```python
from build123d import *

# Parameters (mm, degrees)
F1_DEPTH = 6.0198
F3_DEPTH = 6.0198
F4_R     = 7.62
F5_R     = 1.27


with BuildPart() as f1:
    # F0 (on Top) → F1 (new body)
    with BuildSketch(Plane.XY):
        with BuildLine():
            ThreePointArc((-5.588, -10.4775), (0, 11.8745), (5.588, -10.4775))
            Line((5.588, -10.4775), (5.588, -17.0815))
            Line((5.588, -17.0815), (19.1516, -17.0815))
            Line((19.1516, -17.0815), (19.1516, 21.4503))
            Line((19.1516, 21.4503), (-6.5024, 38.3413))
            ThreePointArc((-6.5024, 38.3413), (-15.638779, 32.001463), (-19.1516, 21.4503))
            Line((-19.1516, 21.4503), (-19.1516, -17.0815))
            Line((-19.1516, -17.0815), (-5.588, -17.0815))
            Line((-5.588, -17.0815), (-5.588, -10.4775))
        make_face()
    extrude(amount=F1_DEPTH)

    # F2 (on face) → F3 (cut, through all)
    with BuildSketch(Plane.XY.offset(6.0198)):
        with BuildLine():
            ThreePointArc((-6.444942, 33.269299), (-11.999418, 28.483341), (-14.0716, 21.4503))
            ThreePointArc((-14.0716, 21.4503), (-11.5316, 18.9103), (-8.9916, 21.4503))
            ThreePointArc((-8.9916, 21.4503), (-7.730957, 25.728955), (-4.35181, 28.640563))
            ThreePointArc((-4.35181, 28.640563), (-3.084008, 32.001498), (-6.444942, 33.269299))
        make_face()
    extrude(amount=-F3_DEPTH, mode=Mode.SUBTRACT)

    # F4
    f4_edges = [f1.edges().sort_by_distance(p)[0] for p in [
        (-6.5024, 38.3413, 3.0099),
        (19.1516, 21.4503, 3.0099),
    ]]
    fillet(f4_edges, radius=F4_R)

    # F5
    f5_edges = [f1.edges().sort_by_distance(p)[0] for p in [
        (-19.1516, -17.0815, 3.0099),
        (-5.588, -17.0815, 3.0099),
        (5.588, -17.0815, 3.0099),
        (19.1516, -17.0815, 3.0099),
        (5.588, -10.4775, 3.0099),
        (-5.588, -10.4775, 3.0099),
    ]]
    fillet(f5_edges, radius=F5_R)


solid = f1.part
```
Geometry check sheet. Reference: the model listing, model coordinates, mm. A direction names the side the tool comes from. Round coordinates to 2 decimals unless told otherwise and drop trailing zeros. Order: outer loops, then holes, each group sorted by start corner. A loop starts at its lowest first (then second) coordinate and runs counter-clockwise, first axis right, second up. Notation, with made-up numbers: (-14, 8) - (12, 8) arc R19 ccw to (12, 36) - close; hole circle Ø3 at (87.25, -16). An arc over 180 degrees is marked (long way). Use a Markdown table: item, result. Add a question column.
1) Thickness scan on line 1 along X through (y, z) = (0, 2.25); line 2 along X through (y, z) = (-7.5, 1.5); line 3 along Y through (x, z) = (-4, 5.25). Record the ranges inside material, lowest first.
2) Section check A-A (y = 0). Record the cut outline in (x, z).
3) Section check D-D (x = 0). Record the cut outline in (y, z), then the cut area to 3 significant figures.
4) Mould release check, pull along Y, two halves, no side actions. Record for faces 4 (the cylindrical face through (18.264, 20.912, 3.052)), 5 (the cylindrical face through (-5.755, -10.585, 3.052)), 6 (the flat face through (0, 17, 0)), 7 (the flat face through (12, -17.082, 3)): released by +Y, released by -Y, zero draft, split by the parting line, or undercut.
5) Gauge pin test, flat ends, axial feed: P1, Ø1, axis at x = 12, z = 2, coming from the +Y side; P2, Ø1.5, axis at x = -3, z = 4.5, coming from the -Y side. Record the tip position at first contact, or that the pin passes through.
6) Set-up check for faces 1 (the cylindrical face through (-5.95, -16.7, 3.05)), 2 (the cylindrical face through (-7.765, 25.676, 3.052)), 3 (the flat face through (-19.152, 3, 3)): record each of +Z, -Z, +X, -X, +Y, -Y from which the full face is reachable in a straight line by a thin tool's end or side.
7) Section check C-C (y = 31). Record the cut outline in (x, z), then the cut area to 3 significant figures.
8) Section check B-B (z = 1.25). Record the cut outline in (x, y).
Established:
| question | item | result |
|---|---|---|
| 1 | line 1 | -19.15 to -11.87, 11.87 to 19.15 |
| 1 | line 2 | -19.15 to -9.21, 9.21 to 19.15 |
| 1 | line 3 | 11.18 to 28.83, 33.08 to 36.59 |
| 2 | outline | (-19.15, 0) - (-11.87, 0) - (-11.87, 6.02) - (-19.15, 6.02) - close; (11.87, 0) - (19.15, 0) - (19.15, 6.02) - (11.87, 6.02) - close |
| 3 | outline | (11.87, 0) - (34.06, 0) - (34.06, 6.02) - (11.87, 6.02) - close |
| 3 | area | 134 mm2 |
| 4 | face 4 | released by +Y |
| 4 | face 5 | undercut |
| 4 | face 6 | zero draft |
| 4 | face 7 | released by -Y |
| 5 | P1 | y = 26.49 |
| 5 | P2 | y = 11.27 |
| 6 | face 1 | +Z, -Z, -Y |
| 6 | face 2 | +Z, -Z |
| 6 | face 3 | +Z, -Z, -X, +Y, -Y |
| 7 | outline | (-16.34, 0) - (-9.88, 0) - (-9.88, 6.02) - (-16.34, 6.02) - close; (-2.86, 0) - (4.65, 0) - (4.65, 6.02) - (-2.86, 6.02) - close |
| 7 | area | 84.1 mm2 |
| 8 | outline | (-19.15, -15.81) arc R1.27 ccw to (-17.88, -17.08) - (-6.86, -17.08) arc R1.27 ccw to (-5.59, -15.81) - (-5.59, -11.21) arc R1.27 ccw to (-6.2, -10.13) arc R11.87 cw (long way) to (6.2, -10.13) arc R1.27 ccw to (5.59, -11.21) - (5.59, -15.81) arc R1.27 ccw to (6.86, -17.08) - (17.88, -17.08) arc R1.27 ccw to (19.15, -15.81) - (19.15, 17.34) arc R7.62 ccw to (15.72, 23.71) - (-3.01, 36.04) arc R7.62 ccw to (-11.52, 35.96) arc R17.6 ccw to (-19.15, 21.45) - close; hole (-14.07, 21.45) arc R2.54 ccw to (-8.99, 21.45) arc R7.89 cw to (-4.35, 28.64) arc R2.54 ccw to (-6.44, 33.27) arc R12.97 ccw to start |
